```python
from build123d import *

# Parameters (mm, degrees)
SKETCH1_R                       = 10.5
BOSS_EXTRUDE1_DEPTH             = 38
SKETCH2_R                       = 6
CUT_EXTRUDE1_DEPTH              = 41.798284278
F_3_9_3_9_DIAMETER_HOLE1_REACH  = 46.668
F_3_9_3_9_DIAMETER_HOLE1_BORE_R = 1.95
F_3_0MM_DOWEL_HOLE1_D           = 3
F_3_0MM_DOWEL_HOLE1_DEPTH       = 6
F_3_0MM_DOWEL_HOLE1_TIP         = 0.901290929
CHAMFER1_SIZE                   = 0.5
F_3_0MM_DOWEL_HOLE2_D           = 3
F_3_0MM_DOWEL_HOLE2_DEPTH       = 8
F_3_0MM_DOWEL_HOLE2_TIP         = 0.901290929


with BuildPart() as part:
    # Sketch1 → Boss-Extrude1 (new body)
    with BuildSketch(Plane(origin=(0, 0, 0), x_dir=(1, 0, 0), z_dir=(0, 1, 0))):
        with Locations(Location((0, 0, 0), (0, 0, 270))):
            Circle(SKETCH1_R)
    extrude(amount=BOSS_EXTRUDE1_DEPTH)

    # Sketch2 → Cut-Extrude1 (cut, through all)
    with BuildSketch(Plane(origin=(0, 38, 0), x_dir=(1, 0, 0), z_dir=(0, 1, 0))):
        with Locations(Location((0, 0, 0), (0, 0, 270))):
            Circle(SKETCH2_R)
    extrude(amount=-CUT_EXTRUDE1_DEPTH, mode=Mode.SUBTRACT)

    # Ø3.9 (3.9) Diameter Hole1 bore → Ø3.9 (3.9) Diameter Hole1 (cut, up to next)
    with BuildSketch(Plane.ZY.offset(10.5), mode=Mode.PRIVATE) as f_3_9_3_9_diameter_hole1_sk1:
        with Locations((0, 30)):
            Circle(F_3_9_3_9_DIAMETER_HOLE1_BORE_R)
    f_3_9_3_9_diameter_hole1_tool1 = extrude(f_3_9_3_9_diameter_hole1_sk1.sketch, amount=-F_3_9_3_9_DIAMETER_HOLE1_REACH, mode=Mode.PRIVATE) & part.part
    f_3_9_3_9_diameter_hole1 = f_3_9_3_9_diameter_hole1_tool1.solids().sort_by_distance((-10.5, 30, 0))[0]
    add(f_3_9_3_9_diameter_hole1, mode=Mode.SUBTRACT)

    # Sketch9 → Ø5.0mm Dowel Hole1 (revolve, cut)
    with BuildSketch(Plane(origin=(-10.5, 30, 0), x_dir=(0, 0, 1), z_dir=(0, 1, 0))):
        Polygon((0, 0), (0, 5.502151548), (2.5, 4), (2.5, 0), align=None)
    f_5_0mm_dowel_hole1 = revolve(axis=Axis((-16.85, 30, 0), (1, 0, 0)), mode=Mode.SUBTRACT)

    # Mirror1: Ø3.9 (3.9) Diameter Hole1, Ø5.0mm Dowel Hole1 across plane
    add(f_3_9_3_9_diameter_hole1.mirror(Plane(origin=(0, 18.5, 0), x_dir=(0, 0, 1), z_dir=(0, -1, 0))), mode=Mode.SUBTRACT)
    add(f_5_0mm_dowel_hole1.mirror(Plane(origin=(0, 18.5, 0), x_dir=(0, 0, 1), z_dir=(0, -1, 0))), mode=Mode.SUBTRACT)

    # Ø3.0mm Dowel Hole1
    with Locations(Plane(origin=(0, 38, 0), x_dir=(1, 0, 0), z_dir=(0, 1, 0))):
        with Locations((8.5, 0), (0, -8.5)):
            Hole(F_3_0MM_DOWEL_HOLE1_D / 2, depth=F_3_0MM_DOWEL_HOLE1_DEPTH)
            with Locations((0, 0, -(F_3_0MM_DOWEL_HOLE1_DEPTH + F_3_0MM_DOWEL_HOLE1_TIP / 2))):  # 118° drill point
                Cone(0, F_3_0MM_DOWEL_HOLE1_D / 2, F_3_0MM_DOWEL_HOLE1_TIP, mode=Mode.SUBTRACT)

    # Chamfer1
    chamfer1_edges = [part.edges().sort_by_distance(p)[0] for p in [
        (0, 38, -6),
    ]]
    chamfer(chamfer1_edges, length=CHAMFER1_SIZE)

    # Ø3.0mm Dowel Hole2
    with Locations(Plane(origin=(0, 38, 0), x_dir=(1, 0, 0), z_dir=(0, 1, 0))):
        with Locations((0, 10.5)):
            Hole(F_3_0MM_DOWEL_HOLE2_D / 2, depth=F_3_0MM_DOWEL_HOLE2_DEPTH)
            with Locations((0, 0, -(F_3_0MM_DOWEL_HOLE2_DEPTH + F_3_0MM_DOWEL_HOLE2_TIP / 2))):  # 118° drill point
                Cone(0, F_3_0MM_DOWEL_HOLE2_D / 2, F_3_0MM_DOWEL_HOLE2_TIP, mode=Mode.SUBTRACT)


solid = part.part
```
Geometry: final body of the model. Coordinates: model frame, mm. A direction names the side the tool comes from. Round coordinates to 2 decimals unless told otherwise and drop trailing zeros. Loops run counter-clockwise (first coordinate to the right, second up) from the corner with the lowest first, then second, coordinate; pieces in that order, holes last. Notation, with made-up numbers: (-10.5, 3.25) -> (46.5, 3.25) arc R6 cw to (46.5, 14.25) -> close; hole circle Ø11 at (-2, 58.25). An arc over 180 degrees is marked (long way). Use one line per item in the form item = value. Start each with the question number.
1) Line query: L1, parallel to X at y = 10, z = 3.5; L2, parallel to X at y = 23, z = 8.25; L3, parallel to Z at x = -2.5, y = 13.5. Output: solid intervals per line, ascending.
2) Section A-A on y = 12.5. Output: boundary loops of the cut face in (x, z).
3) Draft query along Y for faces 1 (the cylindrical face through (0, 34, -9)), 2 (the cylindrical face through (-8.5, 29.9, -2.5)), 3 (the flat face through (-5, 0, 5)). Return one class per face: released by +Y, released by -Y, zero draft, split by the parting line, or undercut.
4) Section C-C on y = 7. Output: boundary loops of the cut face in (x, z).
5) Section B-B on x = -7. Output: boundary loops of the cut face in (y, z), then the cut area to 3 significant figures.
6) First-contact query: P1, Ø1, axis at x = -8, y = 9.5, coming from the +Z side; P2, Ø1.8, axis at x = 0, z = 8.5, coming from the -Y side; P3, Ø3, axis at y = 14, z = 7.5, coming from the -X side; P4, Ø8, axis at x = -5, y = 21, coming from the -Z side. Flat tips, straight axial feed; report the tip coordinate or a pass-through.
7) Access query for faces 4 (the cylindrical face through (-5.977, 6.914, -1.948)), 5 (the flat face through (-5, 38, -5)), 6 (the cylindrical face through (10, 35, 0)). Directions: +Z, -Z, +X, -X, +Y, -Y. A direction counts if a zero-diameter tool reaches every point of the face in a straight line with its end or side. Return the directions, or none.
8) Section D-D on z = 0.5. Give the number of separate pieces and of enclosed holes in the cut face, then the cut area to 3 significant figures.
Response:
q1.L1 = -9.9 to -4.87, 4.87 to 9.9
q1.L2 = -6.5 to 6.5
q1.L3 = -10.2 to -5.45, 5.45 to 10.2
q2.outline = circle Ø21 at (0, 0); hole circle Ø12 at (0, 0)
q3.face_1 = zero draft
q3.face_2 = undercut
q3.face_3 = released by -Y
q4.outline = (-10.2, -2.5) arc R10.5 ccw (long way) to (-10.2, 2.5) -> (-6.5, 2.5) -> (-6.17, 1.95) -> (-5.67, 1.95) arc R6 cw (long way) to (-5.67, -1.95) -> (-6.17, -1.95) -> (-6.5, -2.5) -> close
q5.outline = (0, -7.83) -> (38, -7.83) -> (38, 7.83) -> (0, 7.83) -> close; hole circle Ø5 at (7, 0); hole circle Ø5 at (30, 0)
q5.area = 556 mm^2
q6.P1 = 7.35
q6.P2 = 0
q6.P3 = -8.62
q6.P4 = -10.45
q7.face_4 = -X
q7.face_5 = +Z, -Z, +X, -X, +Y
q7.face_6 = +Y
q8.separate_pieces = 4
q8.enclosed_holes = 0
q8.area = 281 mm^2
